from build123d import *

# Parameters (mm, degrees)
SKETCH1_R      = 69.85
SKETCH1_R_2    = 50.8
SKETCH1_R_3    = 2.57937
EXTRUDE1_DEPTH = 6.35
SKETCH2_R      = 50.8
SKETCH2_R_2    = 47.625
EXTRUDE2_DEPTH = 92.075


with BuildPart() as part:
    # Sketch1 → Extrude1 (new body)
    with BuildSketch(Plane.XY):
        Circle(SKETCH1_R)
        Circle(SKETCH1_R_2, mode=Mode.SUBTRACT)
        with Locations((0, 60.325)):
            Circle(SKETCH1_R_3, mode=Mode.SUBTRACT)
        with Locations((-52.242982483, 30.1625)):
            Circle(SKETCH1_R_3, mode=Mode.SUBTRACT)
        with Locations((-52.242982483, -30.1625)):
            Circle(SKETCH1_R_3, mode=Mode.SUBTRACT)
        with Locations((0, -60.325)):
            Circle(SKETCH1_R_3, mode=Mode.SUBTRACT)
        with Locations((52.242982483, -30.1625)):
            Circle(SKETCH1_R_3, mode=Mode.SUBTRACT)
        with Locations((52.242982483, 30.1625)):
            Circle(SKETCH1_R_3, mode=Mode.SUBTRACT)
    extrude(amount=EXTRUDE1_DEPTH)

    # Sketch2 → Extrude2 (add)
    with BuildSketch(Plane.XY):
        Circle(SKETCH2_R)
        Circle(SKETCH2_R_2, mode=Mode.SUBTRACT)
    extrude(amount=EXTRUDE2_DEPTH)


solid = part.part
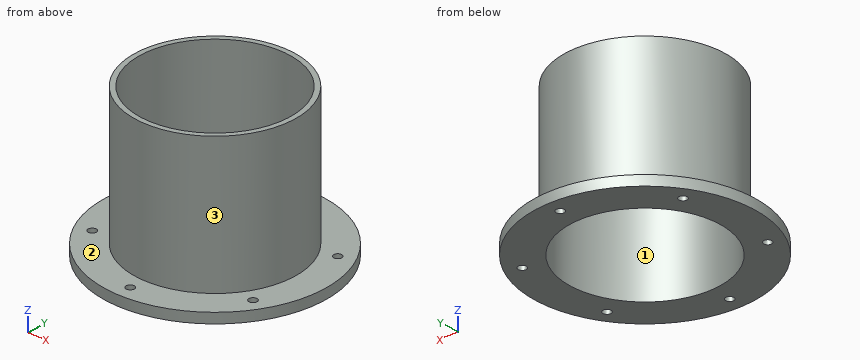
Geometry check sheet. Reference: the model listing, model coordinates, mm. Face numbers are marked on the shaded views. Coordinates: 2 decimals unless noted, no trailing zeros. Order: outer loops, then holes, each group sorted by start corner. A loop starts at its lowest first (then second) coordinate and runs counter-clockwise, first axis right, second up. Notation, with made-up numbers: (23.5, -8.75) -> (36.5, -8.75) arc R32 cw to (36.5, 25.25) -> close; hole circle Ø1 at (26.25, -25.5). An arc over 180 degrees is marked (long way). Use a Markdown table: item, result. Add a question column.
1. Cross-section at C-C (x = 0). Enter the section's corners in (y, z) (3 decimals).
2. Cross-section at D-D (z = 15). Enter the section's corners in (x, y) (3 decimals), and give its area (3 significant figures).
3. Go/stop test with flat-tipped pins: pin 1 Ø8 at (y, z) = (-39.5, 31) entering from +X; pin 2 Ø6.5 at (x, y) = (0, 60.325) entering from +Z; pin 3 Ø3 at (y, z) = (13, 59) entering from +X; pin 4 Ø6 at (x, y) = (52.24, -30.16) entering from -Z. Record where each tip stops, or that it passes through.
4. Cross-section at B-B (x = 41). Enter the section's corners in (y, z) (3 decimals).
5. Cross-section at A-A (y = 0). Enter the section's corners in (x, z) (3 decimals).
6. Material ranges on L1, parallel to Y at x = 0, z = 3 (3 decimals); L2, parallel to X at y = -1, z = 31.5; L3, parallel to Y at x = -1.5, z = 22.5, recorded low to high.
7. Mould release check, pull along Y, two halves, no side actions. Record for the marked faces 1, 2 and 3: pulls with the +Y half, pulls with the -Y half, needs draft (parallel to the pull), parting line crosses it, or undercut.
Filled sheet:
| question | item | result |
|---|---|---|
| 1 | outline | (-69.85, 0) -> (-62.904, 0) -> (-62.904, 6.35) -> (-69.85, 6.35) -> close; (-57.746, 0) -> (-47.625, 0) -> (-47.625, 92.075) -> (-50.8, 92.075) -> (-50.8, 6.35) -> (-57.746, 6.35) -> close; (47.625, 0) -> (57.746, 0) -> (57.746, 6.35) -> (50.8, 6.35) -> (50.8, 92.075) -> (47.625, 92.075) -> close; (62.904, 0) -> (69.85, 0) -> (69.85, 6.35) -> (62.904, 6.35) -> close |
| 2 | outline | circle Ø101.6 at (0, 0); hole circle Ø95.25 at (0, 0) |
| 2 | area | 982 mm2 |
| 3 | pin 1 | x = 36.34 |
| 3 | pin 2 | z = 6.35 |
| 3 | pin 3 | x = 49.48 |
| 3 | pin 4 | z = 0 |
| 4 | outline | (-56.551, 0) -> (-24.231, 0) -> (-24.231, 92.075) -> (-29.994, 92.075) -> (-29.994, 6.35) -> (-56.551, 6.35) -> close; (24.231, 0) -> (56.551, 0) -> (56.551, 6.35) -> (29.994, 6.35) -> (29.994, 92.075) -> (24.231, 92.075) -> close |
| 5 | outline | (-69.85, 0) -> (-47.625, 0) -> (-47.625, 92.075) -> (-50.8, 92.075) -> (-50.8, 6.35) -> (-69.85, 6.35) -> close; (47.625, 0) -> (69.85, 0) -> (69.85, 6.35) -> (50.8, 6.35) -> (50.8, 92.075) -> (47.625, 92.075) -> close |
| 6 | L1 | -69.85 to -62.904, -57.746 to -47.625, 47.625 to 57.746, 62.904 to 69.85 |
| 6 | L2 | -50.79 to -47.61, 47.61 to 50.79 |
| 6 | L3 | -50.78 to -47.6, 47.6 to 50.78 |
| 7 | face 1 | undercut |
| 7 | face 2 | needs draft |
| 7 | face 3 | parting line crosses it |
